The listing builds one solid part. Answer for the finished solid, in the listing's coordinates (mm). A direction names the side the tool comes from. Coordinates: 2 decimals unless noted, no trailing zeros. Order: outer loops, then holes, each group sorted by start corner. A loop starts at its lowest first (then second) coordinate and runs counter-clockwise, first axis right, second up. Notation, with made-up numbers: (46, -16) -> (75, -16) arc R19 cw to (75, -3) -> close; hole circle Ø8 at (83.25, 64). An arc over 180 degrees is marked (long way). Write item = value, one per line.
Autodesk Inventor part; units mm, degrees
ref_plane "YZ Plane" through (0, 0, 0) normal (1, 0, 0) x (0, 1, 0)
ref_plane "XZ Plane" through (0, 0, 0) normal (0, 1, 0) x (-1, 0, 0)
ref_plane "XY Plane" through (0, 0, 0) normal (0, 0, 1) x (1, 0, 0)
sketch "Sketch1" plane through (0, 0, 0) normal (0, 1, 0) x (-1, 0, 0)
  line L0 (0, 0) -> (2.5, 0)
  line L1 (2.5, -18) -> (0, -18)
  line L2 (0, -18) -> (0, 0)
  line L3 (11.5, 2) -> (-1, 2)
  line L4 (-2, 1) -> (-2, -19)
  line L5 (-1, -20) -> (11.5, -20)
  line L6 (12.5, -19) -> (12.5, 1)
  line L7 (2.5, -1.5) -> (3.5, -1.5)
  line L8 (2.5, -16.5) -> (3.5, -16.5)
  line L9 (3.5, -1.5) -> (3.5, -3)
  line L10 (3.5, -3) -> (2.5, -3)
  line L11 (3.5, -16.5) -> (3.5, -15)
  line L12 (3.5, -15) -> (2.5, -15)
  line L13 (2.5, -1.5) -> (2.5, 0)
  line L14 (2.5, -3) -> (2.5, -15)
  line L15 (2.5, -16.5) -> (2.5, -18)
  arc A0 (-1, 2) -> (-2, 1) centre (-1, 1) ccw
  arc A1 (-2, -19) -> (-1, -20) centre (-1, -19) ccw
  arc A2 (11.5, -20) -> (12.5, -19) centre (11.5, -19) ccw
  arc A3 (12.5, 1) -> (11.5, 2) centre (11.5, 1) ccw
  dimension "d0" = 18
  dimension "d1" = 2.5
  dimension "d3" = 2
  dimension "d4" = 2
  dimension "d5" = 2
  dimension "d7" = 1
  dimension "d8" = 15
  dimension "d10" = 1.5
  dimension "d11" = 1.5
  dimension "d12" = 1
sketch "Sketch3" plane through (0, 0, 0) normal (0, 1, 0) x (-1, 0, 0)
  point P0 (0, 0)
extrude "Extrusion1" add sketch "Sketch1" along normal blind 15
sketch "Sketch4" plane through (0, 15, 0) normal (0, 1, 0) x (1, 0, 0)
  point P0 (0, 0)
sketch "Sketch5" plane through (0, 15, 0) normal (0, 1, 0) x (1, 0, 0)
  line L0 (-2.5, 5.75) -> (-3.5, 5.75)
  line L1 (-3.5, 5.75) -> (-3.5, 12.25)
  line L2 (-3.5, 12.25) -> (-2.5, 12.25)
  line L3 (-2.5, 12.25) -> (-2.5, 5.75)
  line L4 (-2.5, 3) -> (-2.5, 15)
  line L5 (-11.5, -2) -> (1, -2)
  point P0 (0, 0)
  dimension "d15" = 1
  dimension "d16" = 6.5
  dimension "d17" = 0
  dimension "d18" = 7.75
extrude "Extrusion2" cut sketch "Sketch5" against normal blind 13
properties part number "clip_fit_prototype"
Q1. The mould has two halves that part along X. Classify faces 1 (the face through (-2.5, 7, -1)), 2 (the face through (-12.5, 7, -9)), 3 (the face through (-7, 15, -9)), 4 (the face through (-3, 7, -1.5)): released by +X, released by -X, zero draft, split by the parting line, or undercut.
The answers:
face_1 = undercut
face_2 = released by -X
face_3 = zero draft
face_4 = undercut
Q2. Each of these flat-tipped pins is pushed along its axis until it touches: pin 1 Ø1.5 at (x, z) = (-7.5, -17) entering from -Y; pin 2 Ø0.5 at (x, z) = (-3, -8) entering from +Y. Where does it stop, or does it pass through?
The answers:
pin_1 = 0
pin_2 = 2
Q3. Find the intervals of material crossed by line 1 along Z through (x, y) = (-3.25, 13); line 2 along X through (y, z) = (2.5, -14.5); line 3 along X through (y, z) = (7.5, -8.25), in increasing order.
The answers:
line_1 = -20 to -16.5, -15 to -12.25, -5.75 to -3, -1.5 to 2
line_2 = -12.5 to -2.5, 0 to 2
line_3 = -12.5 to -3.5, 0 to 2
Q4. Section D-D, the plane z = -17 is taken. Give the vertices of the cut face in (x, y), plus the area to 3 significant figures.
The answers:
outline = (-12.5, 0) -> (-2.5, 0) -> (-2.5, 15) -> (-12.5, 15) -> close; (0, 0) -> (2, 0) -> (2, 15) -> (0, 15) -> close
area = 180 mm2
Q5. A tool of negligible diameter and unlimited length cuts with its end or side. For faces 5 (the face through (-3, 9, -5.75)), 6 (the face through (-12.215, 7.395, -19.699)), 7 (the face through (0, 7, -9)), from which of +Z, -Z, +X, -X, +Y, -Y can it reach the whole face along a straight path? Write none if from no direction.
The answers:
face_5 = +Y
face_6 = -Z, -X, +Y, -Y
face_7 = +Y, -Y
Q6. Section B-B, the plane z = -9 is taken. Give the vertices of the cut face in (x, y).
The answers:
outline = (-12.5, 0) -> (-2.5, 0) -> (-2.5, 2) -> (-3.5, 2) -> (-3.5, 15) -> (-12.5, 15) -> close; (0, 0) -> (2, 0) -> (2, 15) -> (0, 15) -> close
Q7. Section C-C, the plane y = 9 is taken. Give the vertices of the cut face in (x, z), plus the area to 3 significant figures.
The answers:
outline = (-12.5, -19) arc R1 ccw to (-11.5, -20) -> (1, -20) arc R1 ccw to (2, -19) -> (2, 1) arc R1 ccw to (1, 2) -> (-11.5, 2) arc R1 ccw to (-12.5, 1) -> close; hole (-3.5, -16.5) -> (-2.5, -16.5) -> (-2.5, -18) -> (0, -18) -> (0, 0) -> (-2.5, 0) -> (-2.5, -1.5) -> (-3.5, -1.5) -> (-3.5, -3) -> (-2.5, -3) -> (-2.5, -5.75) -> (-3.5, -5.75) -> (-3.5, -12.25) -> (-2.5, -12.25) -> (-2.5, -15) -> (-3.5, -15) -> close
area = 264 mm2
Q8. Section A-A, the plane x = -3 is taken. Give the vertices of the cut face in (y, z).
The answers:
outline = (0, -20) -> (15, -20) -> (15, -16.5) -> (0, -16.5) -> close; (0, -15) -> (15, -15) -> (15, -12.25) -> (2, -12.25) -> (2, -5.75) -> (15, -5.75) -> (15, -3) -> (0, -3) -> close; (0, -1.5) -> (15, -1.5) -> (15, 2) -> (0, 2) -> close
